from build123d import *

# Parameters (mm, degrees)
CYLINDER006_R     = 1.49
CYLINDER006_DEPTH = 10
ARRAY015_Y_COUNT  = 8
ARRAY015_Y_PITCH  = 7.58
BOX051_W          = 10
BOX051_H          = 10
BOX051_DEPTH      = 31
BOX050_W          = 10
BOX050_H          = 10
BOX050_DEPTH      = 30
BOX049_W          = 10
BOX049_H          = 10
BOX049_DEPTH      = 25
BOX048_W          = 10
BOX048_H          = 10
BOX048_DEPTH      = 25
BOX046_W          = 2
BOX046_H          = 80
BOX046_DEPTH      = 18
BOX047_W          = 4
BOX047_H          = 76
BOX047_DEPTH      = 18


with BuildPart() as array015:
    # Cylinder006 → Cylinder006 (new body)
    with BuildSketch(Plane(origin=(143, 6, 13), x_dir=(0, 0, -1), z_dir=(1, 0, 0))):
        Circle(CYLINDER006_R)
    extrude(amount=CYLINDER006_DEPTH)

    # Array015 Y: Array015 ×8


with BuildPart() as array015_1:
    add(array015.part)
    with Locations(*[(0, i * ARRAY015_Y_PITCH, 0) for i in range(1, ARRAY015_Y_COUNT)]):
        add(array015.part)


with BuildPart() as array015_2:
    # Array015 placement: moved
    add(array015_1.part.moved(Location((-30, 7.5, 0))))


with BuildPart() as obj1:
    # Box051 → Box051 (new body)
    with BuildSketch(Plane(origin=(110, 80.8, 0), x_dir=(1, 0, 0), z_dir=(0, 0, 1))):
        with Locations((5, 5)):
            Rectangle(BOX051_W, BOX051_H)
    extrude(amount=BOX051_DEPTH)


with BuildPart() as obj2:
    # Box050 → Box050 (new body)
    with BuildSketch(Plane(origin=(109, -8.8, 0), x_dir=(1, 0, 0), z_dir=(0, 0, 1))):
        with Locations((5, 5)):
            Rectangle(BOX050_W, BOX050_H)
    extrude(amount=BOX050_DEPTH)


with BuildPart() as obj3:
    # Box049 → Box049 (new body)
    with BuildSketch(Plane(origin=(114.8, 78.8, 0), x_dir=(1, 0, 0), z_dir=(0, 0, 1))):
        with Locations((5, 5)):
            Rectangle(BOX049_W, BOX049_H)
    extrude(amount=BOX049_DEPTH)


with BuildPart() as obj4:
    # Box048 → Box048 (new body)
    with BuildSketch(Plane(origin=(114.8, -6.8, 0), x_dir=(1, 0, 0), z_dir=(0, 0, 1))):
        with Locations((5, 5)):
            Rectangle(BOX048_W, BOX048_H)
    extrude(amount=BOX048_DEPTH)


with BuildPart() as obj5:
    # Box046 → Box046 (new body)
    with BuildSketch(Plane(origin=(113, 1, 23), x_dir=(1, 0, 0), z_dir=(0, 0, 1))):
        with Locations((1, 40)):
            Rectangle(BOX046_W, BOX046_H)
    extrude(amount=BOX046_DEPTH)


with BuildPart() as cut051:
    # Box047 → Box047 (new body)
    with BuildSketch(Plane(origin=(113, 3, 23), x_dir=(1, 0, 0), z_dir=(0, 0, 1))):
        with Locations((2, 38)):
            Rectangle(BOX047_W, BOX047_H)
    extrude(amount=BOX047_DEPTH)

    # Fusion008031: union obj5
    add(obj5.part)


with BuildPart() as cut051_1:
    # Fusion008031 placement: moved
    add(cut051.part.moved(Location((0, 0, -19))))

    # Cut047: cut obj4
    add(obj4.part, mode=Mode.SUBTRACT)

    # Cut048: cut obj3
    add(obj3.part, mode=Mode.SUBTRACT)

    # Cut049: cut obj2
    add(obj2.part, mode=Mode.SUBTRACT)

    # Cut050: cut obj1
    add(obj1.part, mode=Mode.SUBTRACT)

    # Cut051: cut Array015
    add(array015_2.part, mode=Mode.SUBTRACT)


solid = cut051_1.part
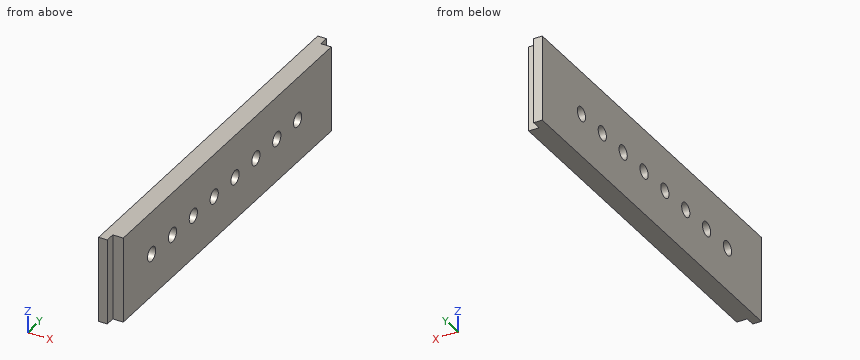
Input: part model. Units: mm. Frame: model coordinates. Coordinates: 2 decimals unless noted, no trailing zeros. Loops run counter-clockwise (first coordinate to the right, second up) from the corner with the lowest first, then second, coordinate; pieces in that order, holes last. Notation, with made-up numbers: (-17.75, 54) -> (30.25, 54) arc R19 ccw to (30.25, 72) -> close; hole circle Ø9 at (84, 59). An arc over 180 degrees is marked (long way). One line per item, written item: value.
(1) Cut plane B-B (y = 36.24). Output: boundary loops of the cut face in (x, z).
Answer below:
outline: (113, 4) -> (117, 4) -> (117, 11.51) -> (113, 11.51) -> close; (113, 14.49) -> (117, 14.49) -> (117, 22) -> (113, 22) -> close
(2) Cut plane A-A (x = 113.65). Give the number of separate pieces and of enclosed holes in the cut face, then the cut area to 3 significant figures.
Answer below:
separate pieces: 1
enclosed holes: 8
area: 1,380 mm2
(3) Cut plane C-C (z = 15.25). Output: boundary loops of the cut face in (x, y).
Answer below:
outline: (113, 1.2) -> (114.8, 1.2) -> (114.8, 3.2) -> (117, 3.2) -> (117, 78.8) -> (114.8, 78.8) -> (114.8, 80.8) -> (113, 80.8) -> close
(4) Ray query, line 1 along Z through (x, y) = (114.05, 51.4); line 2 along Z through (x, y) = (113.3, 42.5); line 3 along Y through (x, z) = (116, 15.5). Return the intervals inside material, ascending.
Answer below:
line 1: z = 4 to 11.51, 14.49 to 22
line 2: z = 4 to 12.31, 13.69 to 22
line 3: y = 3.2 to 78.8
(5) Pin query (flat end, axial travel): pin 1 Ø1.1 at (x, z) = (115.5, 16) entering from +Y; pin 2 Ø4 at (y, z) = (66.56, 13) entering from +X; pin 3 Ø1.6 at (y, z) = (80, 16.5) entering from +X; pin 4 Ø0.7 at (x, z) = (116, 12.5) entering from -Y. Return the tip coordinate at first contact, or that it passes through.
Answer below:
pin 1: stops at y = 78.8
pin 2: stops at x = 117
pin 3: stops at x = 114.8
pin 4: stops at y = 3.2
